```python
from build123d import *

# Parameters (mm, degrees)
SKETCH1_W           = 10
SKETCH1_H           = 10
SKETCH1_W_2         = 8
SKETCH1_H_2         = 8
BOSS_EXTRUDE1_DEPTH = 516
SKETCH2_R           = 2.1
CUT_EXTRUDE1_DEPTH  = 116
SKETCH3_R           = 2.1
CUT_EXTRUDE2_DEPTH  = 5
SKETCH4_R           = 2.1
CUT_EXTRUDE3_DEPTH  = 10


with BuildPart() as part:
    # Sketch1 → Boss-Extrude1 (new body)
    with BuildSketch(Plane.XY):
        with Locations((5, 5)):
            Rectangle(SKETCH1_W, SKETCH1_H)
        with Locations((5, 5)):
            Rectangle(SKETCH1_W_2, SKETCH1_H_2, mode=Mode.SUBTRACT)
    extrude(amount=BOSS_EXTRUDE1_DEPTH)

    # Sketch2 → Cut-Extrude1 (cut)
    with BuildSketch(Plane(origin=(0, 10, 0), x_dir=(1, 0, 0), z_dir=(0, 1, 0))):
        with Locations(Location((5, -5, 0), (0, 0, 270))):
            Circle(SKETCH2_R)
        with Locations(Location((5, -15, 0), (0, 0, 270))):
            Circle(SKETCH2_R)
        with Locations(Location((5, -501, 0), (0, 0, 270))):
            Circle(SKETCH2_R)
        with Locations(Location((5, -511, 0), (0, 0, 270))):
            Circle(SKETCH2_R)
    extrude(amount=-CUT_EXTRUDE1_DEPTH, mode=Mode.SUBTRACT)

    # Sketch3 → Cut-Extrude2 (cut)
    with BuildSketch(Plane.XZ):
        with Locations(Location((5, 308, 0), (0, 0, 270))):
            Circle(SKETCH3_R)
        with Locations(Location((5, 208, 0), (0, 0, 270))):
            Circle(SKETCH3_R)
    extrude(amount=-CUT_EXTRUDE2_DEPTH, mode=Mode.SUBTRACT)

    # Sketch4 → Cut-Extrude3 (cut)
    with BuildSketch(Plane(origin=(10, 0, 0), x_dir=(0, 0, -1), z_dir=(1, 0, 0))):
        with Locations((-416, 5)):
            Circle(SKETCH4_R)
        with Locations((-100, 5)):
            Circle(SKETCH4_R)
        with Locations((-258, 5)):
            Circle(SKETCH4_R)
    extrude(amount=-CUT_EXTRUDE3_DEPTH, mode=Mode.SUBTRACT)


solid = part.part
```
Part model, mm, in its own coordinate system. A direction names the side the tool comes from. Coordinates: 2 decimals unless noted, no trailing zeros. Loops run counter-clockwise (first coordinate to the right, second up) from the corner with the lowest first, then second, coordinate; pieces in that order, holes last. Notation, with made-up numbers: (65.5, 66) - (87.5, 66) arc R31 cw to (87.5, 91) - close; hole circle Ø8 at (88, 81.5). An arc over 180 degrees is marked (long way). Write item = value, one per line. Start each with the question number.
Item 1: Mould opens along X. For faces 1 (the flat face through (1, 5, 254)), 2 (the flat face through (0.5, 5.1, 0)), 3 (the flat face through (10, 5, 254)) say: released by +X, released by -X, zero draft, split by the parting line, or undercut.
Item 2: Cut at A-A, the plane z = 196. Give the cut face in (x, y).
Item 3: Flat gauge pins, fed straight in: pin 1 Ø2.5 at (x, z) = (5, 501) entering from +Y; pin 2 Ø5.5 at (x, z) = (5, 511) entering from +Y; pin 3 Ø4 at (x, z) = (5, 208) entering from -Y. Where does each tip first touch, or does it go through?
Item 4: 3-axis set-ups, long thin cutter, end or side, ignore diameter. For faces 4 (the flat face through (5, 9, 254)), 5 (the flat face through (0.5, 5.1, 516)): which of +Z, -Z, +X, -X, +Y, -Y reach the whole face in a straight line?
Item 5: Wall check: L1, parallel to Y at x = 0.8, z = 100; L2, parallel to X at y = 6.5, z = 435. Give the ranges that are in metal, low to high. Write a range as from..to.
Item 6: Cut at B-B, the plane y = 5. State how many separate pieces and enclosed holes the cut face has, and give its area (3 significant figures).
The answers:
q1.face_1 = undercut
q1.face_2 = zero draft
q1.face_3 = released by +X
q2.outline = (0, 0) - (10, 0) - (10, 10) - (0, 10) - close; hole (1, 1) - (9, 1) - (9, 9) - (1, 9) - close
q3.pin_1 = through
q3.pin_2 = 10
q3.pin_3 = 9
q4.face_4 = +Z, -Z
q4.face_5 = +Z, +X, -X, +Y, -Y
q5.L1 = 0..2.9, 7.1..10
q5.L2 = 0..1, 9..10
q6.separate_pieces = 8
q6.enclosed_holes = 0
q6.area = 1,010 mm2
